from build123d import *
from build123d.topology import SkipClean

# Parameters (mm, degrees)
SKETCH1_W           = 72.26
SKETCH1_H           = 24
BOSS_EXTRUDE1_DEPTH = 36.13
CUT_EXTRUDE1_DEPTH  = 82.675482857
SKETCH3_R           = 3.39
CUT_EXTRUDE2_DEPTH  = 57.451340108
SKETCH4_R           = 6.42
CUT_EXTRUDE3_DEPTH  = 10.42
CUT_EXTRUDE4_DEPTH  = 71.105305077


with BuildPart() as part:
    # Sketch1 → Boss-Extrude1 (new, symmetric)
    with BuildSketch(Plane.XY):
        Rectangle(SKETCH1_W, SKETCH1_H)
    boss_extrude1 = extrude(amount=BOSS_EXTRUDE1_DEPTH, both=True)

    # Sketch2 → Cut-Extrude1 (cut, through all)
    with BuildSketch(Plane.XY.offset(36.13)):
        with BuildLine():
            Line((-16, -12), (16, -12))
            ThreePointArc((16, -12), (0, 4), (-16, -12))
        make_face()
    cut_extrude1 = extrude(amount=-CUT_EXTRUDE1_DEPTH, mode=Mode.SUBTRACT)

    # Sketch3 → Cut-Extrude2 (cut, through all)
    with BuildSketch(Plane(origin=(0, 12, 0), x_dir=(1, 0, 0), z_dir=(0, 1, 0))):
        with Locations(Location((-26.0675, 23.43, 0), (0, 0, 270))):
            Circle(SKETCH3_R)
        with Locations(Location((26.0675, -23.43, 0), (0, 0, 90))):
            Circle(SKETCH3_R)
    cut_extrude2 = extrude(amount=-CUT_EXTRUDE2_DEPTH, mode=Mode.SUBTRACT)

    # Mirror2: Boss-Extrude1, Cut-Extrude1, Cut-Extrude2 across plane
    with SkipClean():  # the faces are left unmerged after this step: merging them gives an invalid solid
        add(boss_extrude1.mirror(Plane(origin=(-36.13, -12, 36.13), x_dir=(0, 0, 1), z_dir=(0, 1, 0))))
        add(cut_extrude1.mirror(Plane(origin=(-36.13, -12, 36.13), x_dir=(0, 0, 1), z_dir=(0, 1, 0))), mode=Mode.SUBTRACT)
        add(cut_extrude2.mirror(Plane(origin=(-36.13, -12, 36.13), x_dir=(0, 0, 1), z_dir=(0, 1, 0))), mode=Mode.SUBTRACT)
    add(part.part.scale(1), mode=Mode.REPLACE)  # the faces are merged on a copy

    # Sketch4 → Cut-Extrude3 (cut)
    with BuildSketch(Plane(origin=(0, 12, 0), x_dir=(1, 0, 0), z_dir=(0, 1, 0))):
        with Locations(Location((-26.0675, 23.43, 0), (0, 0, 270))):
            Circle(SKETCH4_R)
        with Locations(Location((26.0675, -23.43, 0), (0, 0, 90))):
            Circle(SKETCH4_R)
    extrude(amount=-CUT_EXTRUDE3_DEPTH, mode=Mode.SUBTRACT)

    # Sketch5 → Cut-Extrude4 (cut, through all)
    with BuildSketch(Plane(origin=(0, 12, 0), x_dir=(1, 0, 0), z_dir=(0, 1, 0))):
        Polygon((-20.13, -36.13), (-36.13, 8.87), (-36.13, -36.13), align=None)
        Polygon((36.13, 36.13), (36.13, -8.87), (20.13, 36.13), align=None)
    extrude(amount=-CUT_EXTRUDE4_DEPTH, mode=Mode.SUBTRACT)


solid = part.part
Work out the finished part from the listing and answer in its coordinate system (mm). A direction names the side the tool comes from. Give positions to 0.01 mm unless a question says otherwise; leave off trailing zeros. Order: outer loops, then holes, each group sorted by start corner. A loop starts at its lowest first (then second) coordinate and runs counter-clockwise, first axis right, second up. Notation, with made-up numbers: (-33.5, -16) -> (-12.5, -16) arc R27 ccw to (-12.5, 8) -> close; hole circle Ø6 at (-19.75, 15.5). An arc over 180 degrees is marked (long way). One line per item, written item: value.
Item 1: Find section C-C, the plane z = 24.5. Give the vertices of the cut face in (x, y), plus the area to 3 significant figures.
Answer sheet:
outline: (-24.27, -36) -> (22.85, -36) -> (22.85, 1.58) -> (19.74, 1.58) -> (19.74, 12) -> (-24.27, 12) -> close; (29.28, -36) -> (36.13, -36) -> (36.13, 12) -> (32.4, 12) -> (32.4, 1.58) -> (29.28, 1.58) -> close; hole circle Ø32 at (0, -12)
area: 1,720 mm²
Item 2: Flat-ended cylindrical pins translate along their axes: P1, Ø10.5, axis at x = -26.07, z = -23.43, coming from the +Y side; P2, Ø6, axis at y = -27, z = 1, coming from the +X side; P3, Ø1.5, axis at y = -28, z = -27, coming from the +X side. Find the tip coordinate at first contact, or state that the pin passes through.
Answer sheet:
P1: y = 1.58
P2: x = 34.4
P3: x = 23.64
Item 3: Find section A-A, the plane y = -24. Give the vertices of the cut face in (x, z), plus the area to 3 significant figures.
Answer sheet:
outline: (-36.13, -36.13) -> (-10.58, -36.13) -> (-10.58, 36.13) -> (-20.13, 36.13) -> (-36.13, -8.87) -> close; (10.58, -36.13) -> (20.13, -36.13) -> (36.13, 8.87) -> (36.13, 36.13) -> (10.58, 36.13) -> close; hole circle Ø6.78 at (-26.07, -23.43); hole circle Ø6.78 at (26.07, 23.43)
area: 2,900 mm²
Item 4: Straight lines are drawn through the part: probe 1 along X at (y, z) = (-13, -23); probe 2 along Y at (x, z) = (0, -14.5); probe 3 along X at (y, z) = (-2, -5.5). For each, find the intervals that lie inside material, in ascending order.
Answer sheet:
probe 1: -36.13 to -29.43, -22.7 to -15.97, 15.97 to 24.8
probe 2: -36 to -28, 4 to 12
probe 3: -34.93 to -12.49, 12.49 to 31.02
Item 5: Determine the mould class of faces 3 (the flat face through (20, -12, 36.13)), 4 (the cylindrical face through (-22.706, -17.473, -23.871)), 5 (the flat face through (-36.13, -12, -22)) for opening direction X: released by +X, released by -X, zero draft, split by the parting line, or undercut.
Answer sheet:
face 3: zero draft
face 4: undercut
face 5: released by -X
Item 6: A tool of negligible diameter and unlimited length cuts with its end or side. For faces 1 (the flat face through (-29, 1.58, -21)), 2 (the cylindrical face through (22.706, -17.473, 23.871)), from which of +Z, -Z, +X, -X, +Y, -Y can it reach the whole face along a straight path? Write none if from no direction.
Answer sheet:
face 1: +Y
face 2: +Y, -Y
Item 7: Find section D-D, the plane z = 6.5. Give the vertices of the cut face in (x, y), plus the area to 3 significant figures.
Answer sheet:
outline: (-30.67, -36) -> (35.29, -36) -> (35.29, 12) -> (-30.67, 12) -> close; hole circle Ø32 at (0, -12)
area: 2,360 mm²
Item 8: Find section B-B, the plane x = 0. Give the vertices of the cut face in (y, z).
Answer sheet:
outline: (-36, -36.13) -> (-28, -36.13) -> (-28, 36.13) -> (-36, 36.13) -> close; (4, -36.13) -> (12, -36.13) -> (12, 36.13) -> (4, 36.13) -> close
